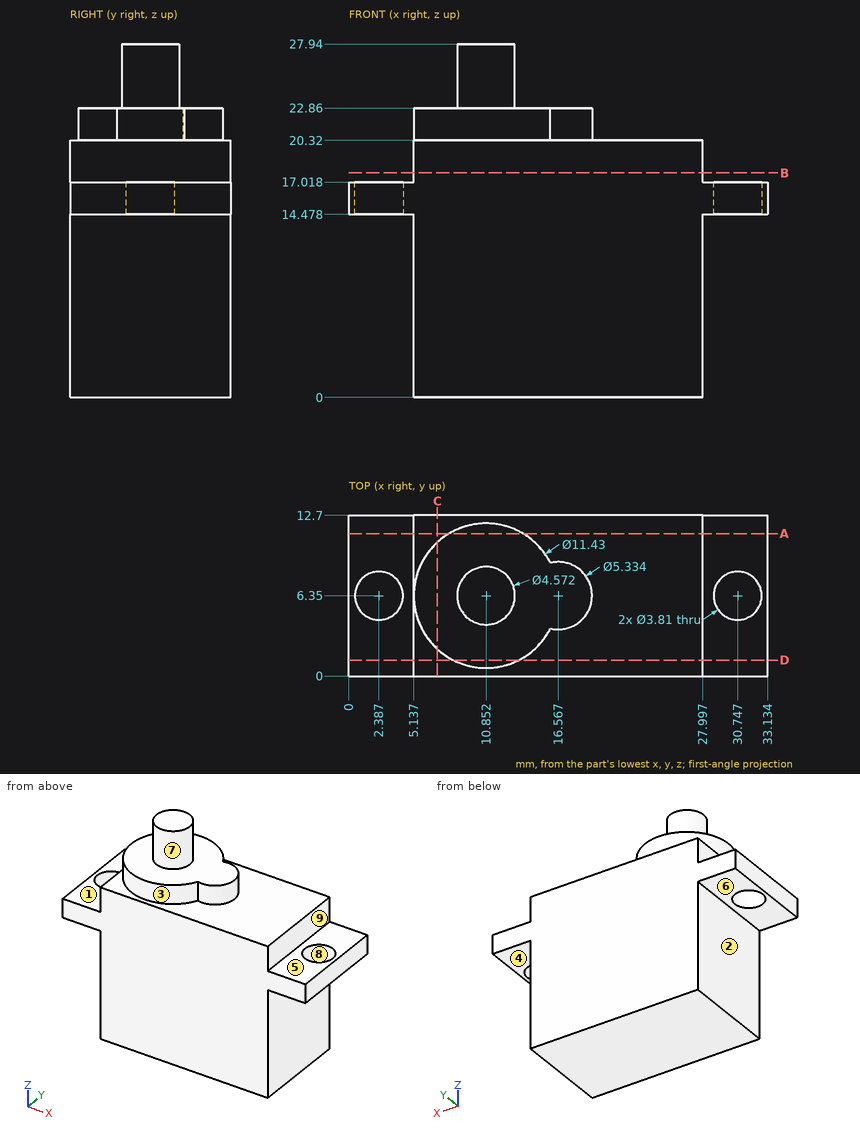
Here's the drawing with two shaded views (mm, measured from the low corner). I have some questions. A direction names the side the tool comes from. Give positions to 0.01 mm unless a question says otherwise; leave off trailing zeros. Write each loop counter-clockwise with the first axis right and the second up, starting at its lowest first coordinate (ties: lowest second). Pieces come first, ordered by that corner, then holes. Notation, with made-up numbers: (76.5, -39.75) -> (81.5, -39.75) arc R27 ccw to (81.5, -0.75) -> close; hole circle Ø5 at (5, -17). An arc over 180 degrees is marked (long way). One line per item, written item: value.
Q1. Which directions (+Z, -Z, +X, -X, +Y, -Y) give clear straight access to the entire face, cutting with the end or side of a thin tool? Please do the marked faces 1, 2, 3, 4 and 5.
Results found:
face 1: +Z, -X, +Y, -Y
face 2: -Z, -X, +Y, -Y
face 3: +Z
face 4: -Z, +X, +Y, -Y
face 5: +Z, +X, +Y, -Y
Q2. We'd pull the mould along X, two halves only. Please class the marked faces 6, 7, 8 and 9: +X half, -X half, draft (parallel to the pull), parting line (faces both ways), or undercut.
Results found:
face 6: draft
face 7: parting line
face 8: undercut
face 9: +X half
Q3. Imagine slicing it at A-A on y = 11.25. Please give me the cut outline in (x, z), and give its area (3 significant figures).
Results found:
outline: (0, 14.48) -> (5.14, 14.48) -> (5.14, 0) -> (28, 0) -> (28, 14.48) -> (33.13, 14.48) -> (33.13, 17.02) -> (28, 17.02) -> (28, 20.32) -> (13.79, 20.32) -> (13.79, 22.86) -> (7.91, 22.86) -> (7.91, 20.32) -> (5.14, 20.32) -> (5.14, 17.02) -> (0, 17.02) -> close
area: 506 mm^2
Q4. For P1, Ø4, axis at y = 5.5, z = 15.5, coming from the -X side; P2, Ø4.5, axis at x = 30.75, y = 6.35, coming from the +Z side; P3, Ø6.5, axis at y = 5, z = 6.5, coming from the +X side; P4, Ø2.5, axis at y = 3.5, z = 18.5, coming from the -X side, each with a flat end and sliding along its axis, tell me the tip position at first contact or that it passes through.
Results found:
P1: stops at x = 0
P2: stops at z = 17.02
P3: stops at x = 28
P4: stops at x = 5.14
Q5. Imagine slicing it at D-D on y = 1.25. Please give me the cut outline in (x, z).
Results found:
outline: (0, 14.48) -> (5.14, 14.48) -> (5.14, 0) -> (28, 0) -> (28, 14.48) -> (33.13, 14.48) -> (33.13, 17.02) -> (28, 17.02) -> (28, 20.32) -> (13.43, 20.32) -> (13.43, 22.86) -> (8.27, 22.86) -> (8.27, 20.32) -> (5.14, 20.32) -> (5.14, 17.02) -> (0, 17.02) -> close
Q6. Imagine slicing it at B-B on z = 17.75. Please give me the cut outline in (x, y).
Results found:
outline: (5.14, 0) -> (28, 0) -> (28, 12.7) -> (5.14, 12.7) -> close
Q7. Imagine slicing it at C-C on x = 7. Please give me the cut outline in (y, z).
Results found:
outline: (0, 0) -> (12.7, 0) -> (12.7, 20.32) -> (10.57, 20.32) -> (10.57, 22.86) -> (2.13, 22.86) -> (2.13, 20.32) -> (0, 20.32) -> close
Q8. Please list where these lines run through material, in increasing order: line 1 (X direction, y = 6.25, z = 16.75); line 2 (Z direction, x = 13, y = 11); line 3 (Z direction, x = 21, y = 11.75). Write a range as [from, to].
Results found:
line 1: x = [0, 0.48], [4.29, 28.84], [32.65, 33.13]
line 2: z = [0, 22.86]
line 3: z = [0, 20.32]
